Study the drawing (mm; zero at the part's minimum x, y, z) and answer. A direction names the side the tool comes from. Coordinates: 2 decimals unless noted, no trailing zeros. Order: outer loops, then holes, each group sorted by start corner. A loop starts at its lowest first (then second) coordinate and runs counter-clockwise, first axis right, second up. Notation, with made-up numbers: (0.5, -4.5) -> (11.5, -4.5) arc R13 ccw to (11.5, 1.5) -> close; hole circle Ø3 at (31, -24). An arc over 180 degrees is marked (long way). Write each question's results on one line, items separated by ' | '. Start each with the question number.
(1) The part is cut by section D-D, the plane x = 31.5. Give the vertices of the cut face in (y, z) (1 decimal), then the cut area to 3 significant figures.
(2) The part is cut by section B-B, the plane z = 18.25. Give the vertices of the cut face in (x, y).
(3) The part is cut by section A-A, the plane x = 10. Give the vertices of the cut face in (y, z) (1 decimal).
(4) A tool of negligible diameter and unlimited length cuts with its end or side. For the marked faces 1 and 2, from which of +Z, -Z, +X, -X, +Y, -Y can it reach the whole face along a straight path? Write none if from no direction.
(5) Given pin 1 (4 mm diameter, centred on x = 37, z = 16, fed in from +Y); pin 2 (3 mm diameter, centred on x = 15.5, z = 10, fed in from -Y); pin 3 (6 mm diameter, centred on y = 4.5, z = 8, fed in from +X), each flat-ended and moving along its own axis, determine where each tip first touches the part or whether it passes through.
(6) Straight lines are drawn through the part: L1, parallel to Z at x = 24, y = 3 (1 decimal); L2, parallel to X at y = 15.25, z = 2 (1 decimal); L3, parallel to Y at x = 18, z = 3.5 (1 decimal). For each, find the intervals that lie inside material, in ascending order.
(7) The part is cut by section C-C, the plane z = 2.75. Give the vertices of the cut face in (x, y) (1 decimal), then the cut area to 3 significant figures.
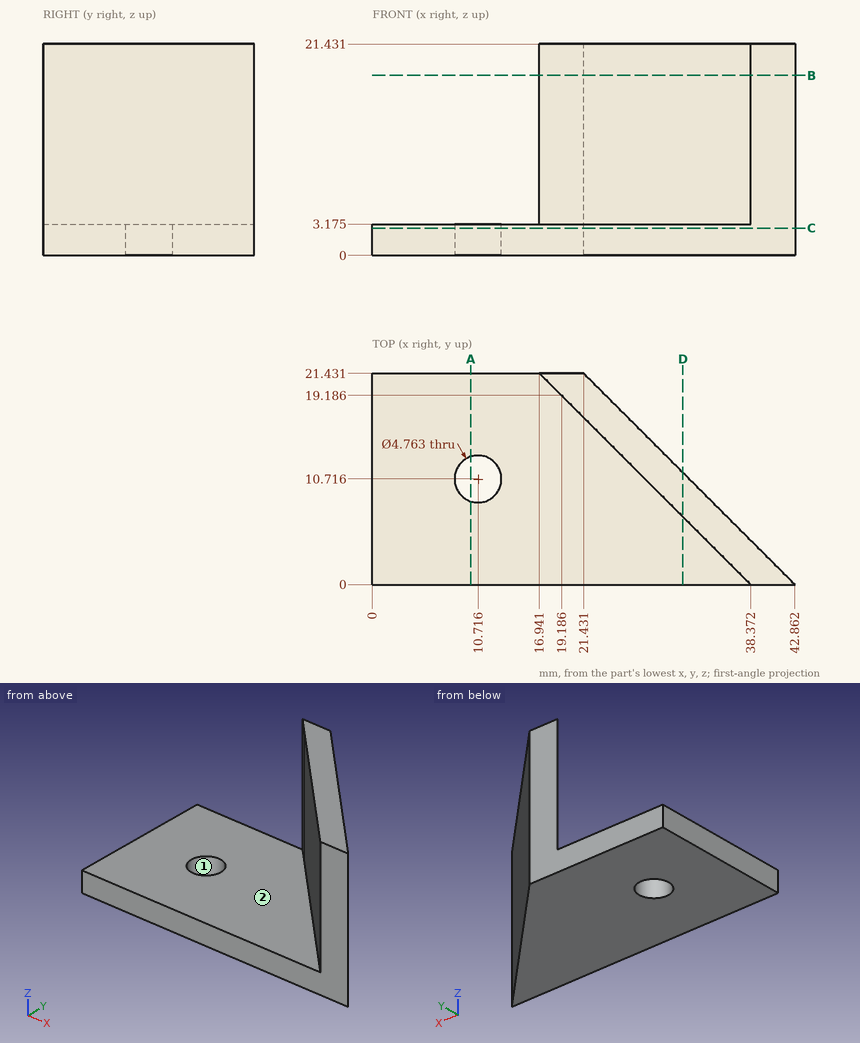
Established:
1) outline: (0, 0) -> (11.4, 0) -> (11.4, 21.4) -> (6.9, 21.4) -> (6.9, 3.2) -> (0, 3.2) -> close | area: 118 mm^2
2) outline: (16.94, 21.43) -> (38.37, 0) -> (42.86, 0) -> (21.43, 21.43) -> close
3) outline: (0, 0) -> (8.4, 0) -> (8.4, 3.2) -> (0, 3.2) -> close; (13, 0) -> (21.4, 0) -> (21.4, 3.2) -> (13, 3.2) -> close
4) face 1: +Z, -Z | face 2: +Z, -X, -Y
5) pin 1: stops at y = 7.86 | pin 2: stops at y = 21.37 | pin 3: stops at x = 41.36
6) L1: z = 0 to 3.2 | L2: x = 0 to 27.6 | L3: y = 20.4 to 21.4
7) outline: (0, 0) -> (42.9, 0) -> (21.4, 21.4) -> (0, 21.4) -> close; hole circle Ø4.8 at (10.7, 10.7) | area: 671 mm^2
